Source: CAD feature listing. Evaluate the final solid. Frame: model axes, mm. Face numbers are marked on the shaded views. A direction names the side the tool comes from. Round coordinates to 2 decimals unless told otherwise and drop trailing zeros. Loops run counter-clockwise (first coordinate to the right, second up) from the corner with the lowest first, then second, coordinate; pieces in that order, holes last. Notation, with made-up numbers: (84, 52) - (97, 52) arc R20 ccw to (97, 76) - close; hole circle Ø3 at (33.5, 27.25). An arc over 180 degrees is marked (long way). Use CSV: the item, a comma, the result in double quotes. Start each with the question number.
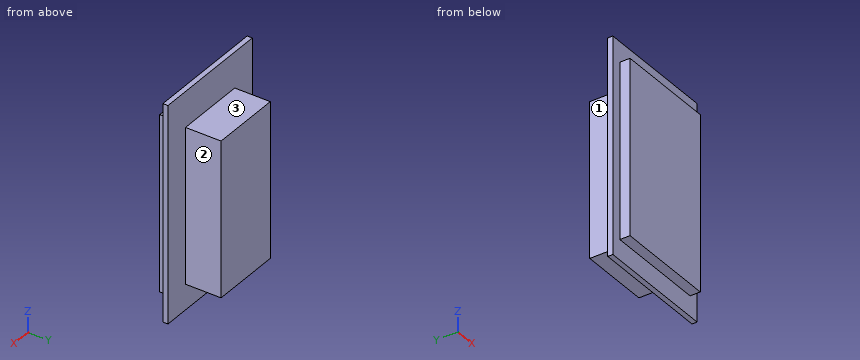
Autodesk Inventor part; units mm, degrees
ref_plane "YZ Plane" through (0, 0, 0) normal (1, 0, 0) x (0, 1, 0)
ref_plane "XZ Plane" through (0, 0, 0) normal (0, 1, 0) x (-1, 0, 0)
ref_plane "XY Plane" through (0, 0, 0) normal (0, 0, 1) x (1, 0, 0)
sketch "スケッチ1" plane through (0, 0, 0) normal (0, 1, 0) x (-1, 0, 0)
  line L0 (12, -21.25) -> (-12, -21.25)
  line L1 (-12, -21.25) -> (-12, 21.25)
  line L2 (-12, 21.25) -> (12, 21.25)
  line L3 (12, 21.25) -> (12, -21.25)
  line L4 (12, -21.25) -> (-12, 21.25) construction
  line L5 (-12, -21.25) -> (12, 21.25) construction
  point P0 (0, 0)
  dimension "d0" = 24
  dimension "d1" = 42.5
extrude "押し出し1" add sketch "スケッチ1" along normal blind 1
sketch "スケッチ2" plane through (0, 0, 0) normal (0, -1, 0) x (1, 0, 0)
  line L0 (-12, 21.25) -> (12, 21.25)
  line L1 (-12, -21.25) -> (-12, 21.25)
  line L2 (12, -21.25) -> (-12, -21.25)
  line L3 (12, 21.25) -> (12, -21.25)
  line L4 (-10, 17.25) -> (10, 17.25)
  line L5 (10, 17.25) -> (10, -17.25)
  line L6 (10, -17.25) -> (-10, -17.25)
  line L7 (-10, -17.25) -> (-10, 17.25)
  point P0 (0, 0)
  dimension "d4" = 4
  dimension "d5" = 4
  dimension "d6" = 2
  dimension "d7" = 2
extrude "押し出し2" add sketch "スケッチ2" along normal blind 2 contours L4 L5 L6 L7
sketch "スケッチ3" plane through (0, 1, 0) normal (0, 1, 0) x (1, 0, 0)
  line L0 (7, -14.25) -> (-7, -14.25)
  line L1 (-7, -14.25) -> (-7, 16.25)
  line L2 (-7, 16.25) -> (7, 16.25)
  line L3 (7, 16.25) -> (7, -14.25)
  line L4 (-12, -21.25) -> (12, -21.25)
  line L5 (12, 21.25) -> (-12, 21.25)
  line L6 (12, -21.25) -> (12, 21.25)
  line L7 (-12, 21.25) -> (-12, -21.25)
  point P0 (0, 0)
  dimension "d10" = 7
  dimension "d11" = 5
  dimension "d12" = 5
  dimension "d13" = 5
extrude "押し出し3" add sketch "スケッチ3" along normal blind 7 contours L0 L1 L2 L3
properties part number "HW-069"
1. Section query C-C on y = 6.25. Return the cut outline in (x, z).
2. Section query A-A on x = -3.5. Return the cut outline in (y, z), and give its area (3 significant figures).
3. Contact query for flat-ended pins moving along their axis: P1, Ø5, axis at y = 6, z = -4.5, coming from the +X side; P2, Ø3.5, axis at x = 0.5, y = 5.5, coming from the +Z side; P3, Ø0.6, axis at x = -0.5, y = -1, coming from the +Z side; P4, Ø2, axis at x = 9, y = 5, coming from the -Z side. Output: stop coordinate, or through.
4. Reachability of the marked faces 1, 2 and 3 from +Z, -Z, +X, -X, +Y, -Y: full face, straight path, thin tool, end or side. Return the list, or none.
5. Section query D-D on z = -7. Return the cut outline in (x, y), and give its area (3 significant figures).
6. Section query B-B on z = 15. Return the cut outline in (x, y), and give its area (3 significant figures).
7. Line query: line 1 along Y through (x, z) = (-8.25, 0); line 2 along X through (y, z) = (2.5, -2); line 3 along Z through (x, y) = (-2.75, 3.25). Output: solid intervals per line, ascending.
Values:
1,outline,"(-7, -16.25) - (7, -16.25) - (7, 14.25) - (-7, 14.25) - close"
2,outline,"(-2, -17.25) - (0, -17.25) - (0, -21.25) - (1, -21.25) - (1, -16.25) - (8, -16.25) - (8, 14.25) - (1, 14.25) - (1, 21.25) - (0, 21.25) - (0, 17.25) - (-2, 17.25) - close"
2,area,"325 mm^2"
3,P1,"stops at x = 7"
3,P2,"stops at z = 14.25"
3,P3,"stops at z = 17.25"
3,P4,"passes through"
4,face 1,"+Z, -Z, -X, +Y"
4,face 2,"+Z, -Z, +X, +Y"
4,face 3,"+Z, +X, -X, +Y"
5,outline,"(-12, 0) - (-10, 0) - (-10, -2) - (10, -2) - (10, 0) - (12, 0) - (12, 1) - (7, 1) - (7, 8) - (-7, 8) - (-7, 1) - (-12, 1) - close"
5,area,"162 mm^2"
6,outline,"(-12, 0) - (-10, 0) - (-10, -2) - (10, -2) - (10, 0) - (12, 0) - (12, 1) - (-12, 1) - close"
6,area,"64.0 mm^2"
7,line 1,"y = -2 to 1"
7,line 2,"x = -7 to 7"
7,line 3,"z = -16.25 to 14.25"
